from build123d import *

# Parameters (mm, degrees)
F0_W     = 60
F0_H     = 70
F0_R     = 2.5
F1_DEPTH = 5
F2_W     = 5
F2_H     = 130
F2_H_2   = 70
F3_DEPTH = 100
F5_DEPTH = 25
F6_W     = 15
F6_H     = 50
F6_W_2   = 5
F7_DEPTH = 5
F9_D     = 5
F9_DEPTH = 40


with BuildPart() as f1:
    # F0 (on Front) → F1 (new body)
    with BuildSketch(Plane.XZ):
        Rectangle(F0_W, F0_H)
        with Locations((-22, -21)):
            Circle(F0_R, mode=Mode.SUBTRACT)
        with Locations((22, -21)):
            Circle(F0_R, mode=Mode.SUBTRACT)
        with Locations((-22, 0)):
            Circle(F0_R, mode=Mode.SUBTRACT)
        with Locations((-22, 21)):
            Circle(F0_R, mode=Mode.SUBTRACT)
        with Locations((22, 0)):
            Circle(F0_R, mode=Mode.SUBTRACT)
        with Locations((22, 21)):
            Circle(F0_R, mode=Mode.SUBTRACT)
    extrude(amount=F1_DEPTH)

    # F2 (on face) → F3 (join)
    with BuildSketch(Plane.XZ.offset(5)):
        with Locations((-7.5, -100)):
            Rectangle(F2_W, F2_H)
        with Locations((-7.5, 0)):
            Rectangle(F2_W, F2_H_2)
        with Locations((7.5, 0)):
            Rectangle(F2_W, F2_H_2)
        with Locations((7.5, -100)):
            Rectangle(F2_W, F2_H)
    extrude(amount=F3_DEPTH)

    # F4 (on face) → F5 (cut)
    with BuildSketch(Plane.YZ.offset(10)):
        Polygon((-105, -15), (-55, 35), (-105, 35), align=None)
        Polygon((-5, -165), (-5, -35), (-55, -85), (-55, -165), align=None)
    extrude(amount=-F5_DEPTH, mode=Mode.SUBTRACT)

    # F6 (on face) → F7 (join)
    with BuildSketch(Plane(origin=(0, 0, -165), x_dir=(1, 0, 0), z_dir=(0, 0, -1))):
        with Locations((-2.5, 80)):
            Rectangle(F6_W, F6_H)
        with Locations((7.5, 80)):
            Rectangle(F6_W_2, F6_H)
    extrude(amount=F7_DEPTH)

    # F9
    with Locations(Plane(origin=(0, 0, -170), x_dir=(1, 0, 0), z_dir=(0, 0, -1))):
        with Locations((0, 90), (0, 70)):
            Hole(F9_D / 2, depth=F9_DEPTH)


solid = f1.part
Can you work these out from the model? Positions are in its coordinate system, mm. A direction names the side the tool comes from. Give positions to 0.01 mm unless a question says otherwise; leave off trailing zeros. Loops run counter-clockwise (first coordinate to the right, second up) from the corner with the lowest first, then second, coordinate; pieces in that order, holes last. Notation, with made-up numbers: (-20.75, 28.25) - (-0.75, 28.25) arc R11 cw to (-0.75, 45.25) - close; hole circle Ø7 at (44, 42). An arc over 180 degrees is marked (long way). Return JSON: item names as keys, results as strings.
1. For faces 4 (the face through (0, -5, 0)), 5 (the face through (18, -5, 0)), 6 (the face through (-10, -65, -43)), 7 (the face through (-7, -55, -127)), 8 (the face through (-5, -65, -44)), which set-ups out of +Z, -Z, +X, -X, +Y, -Y let a thin tool reach every point of the face, with its end or its side?
Output values:
{"face 4": "+Z, -Z, -Y", "face 5": "+Z, -Z, +X, -Y", "face 6": "+Z, -Z, -X, -Y", "face 7": "-Z, +X, -X, +Y", "face 8": "+Z, -Y"}
2. I'm going to push flat-ended pins straight in: pin 1 Ø10 at (y, z) = (-21, -0.5) entering from +X; pin 2 Ø3 at (x, y) = (1, -84.5) entering from +Z; pin 3 Ø6.5 at (x, z) = (22, 21) entering from -Y. Where does each tip first touch, or does it pass through?
Output values:
{"pin 1": "stops at x = 10", "pin 2": "stops at z = -165", "pin 3": "stops at y = -5"}
3. I want a section at D-D on z = -63. Please give me the cut outline in (x, y), and give its area (3 significant figures).
Output values:
{"outline": "(-10, -105) - (-5, -105) - (-5, -33) - (-10, -33) - close; (5, -105) - (10, -105) - (10, -33) - (5, -33) - close", "area": "720 mm²"}
4. I want a section at B-B on z = -21. Please give me the cut outline in (x, y).
Output values:
{"outline": "(-30, -5) - (-24.5, -5) - (-24.5, 0) - (-30, 0) - close; (-19.5, -5) - (-10, -5) - (-10, -105) - (-5, -105) - (-5, -5) - (5, -5) - (5, -105) - (10, -105) - (10, -5) - (19.5, -5) - (19.5, 0) - (-19.5, 0) - close; (24.5, -5) - (30, -5) - (30, 0) - (24.5, 0) - close"}
5. I want a section at A-A on x = -22. Please give me the cut outline in (y, z), and give its area (3 significant figures).
Output values:
{"outline": "(-5, -35) - (0, -35) - (0, -23.5) - (-5, -23.5) - close; (-5, -18.5) - (0, -18.5) - (0, -2.5) - (-5, -2.5) - close; (-5, 2.5) - (0, 2.5) - (0, 18.5) - (-5, 18.5) - close; (-5, 23.5) - (0, 23.5) - (0, 35) - (-5, 35) - close", "area": "275 mm²"}
6. I want a section at C-C on y = -90. Please give me the cut outline in (x, z).
Output values:
{"outline": "(-10, -170) - (-2.5, -170) - (-2.5, -165) - (-5, -165) - (-5, 0) - (-10, 0) - close; (2.5, -170) - (10, -170) - (10, 0) - (5, 0) - (5, -165) - (2.5, -165) - close"}
7. If I drill on line 1 (Z direction, x = -22, y = -3); line 2 (X direction, y = -35, z = 18); line 3 (X direction, y = -90, z = -168), over which ranges is the centre line in solid material (lowest first)?
Output values:
{"line 1": "z = -35 to -23.5, -18.5 to -2.5, 2.5 to 18.5, 23.5 to 35", "line 2": "x = -10 to -5, 5 to 10", "line 3": "x = -10 to -2.5, 2.5 to 10"}
8. We'd pull the mould along Z, two halves only. Please class faces 1 (the face through (10, -65, -43)), 2 (the face through (0, -80, -165)), 3 (the face through (-24.5, -2.5, 0.1)): +Z half, -Z half, draft (parallel to the pull), parting line (faces both ways), or undercut.
Output values:
{"face 1": "draft", "face 2": "+Z half", "face 3": "undercut"}
